Build history of the part. All positions in model axes, mm. A direction names the side the tool comes from. Give positions to 0.01 mm unless a question says otherwise; leave off trailing zeros. Loops run counter-clockwise (first coordinate to the right, second up) from the corner with the lowest first, then second, coordinate; pieces in that order, holes last. Notation, with made-up numbers: M -35,52.5 L -13,52.5 A35 cw -13,85.5 Z; hole C 67.25,-39 d10. An arc over 180 degrees is marked long. Answer in a Markdown table with one row per item. Add a question column.
```python
from build123d import *

# Parameters (mm, degrees)
BOSS_EXTRUDE1_DEPTH       = 40
REVOLVE1_START            = -44.95139953
REVOLVE1_OUTLINE_R        = 13.5
REVOLVE1_DEPTH            = 30.829897511
M18_CLEARANCE_HOLE1_D     = 20
M18_CLEARANCE_HOLE1_DEPTH = 25
SKETCH9_W                 = 1.6
SKETCH9_H                 = 27
CUT_EXTRUDE4_DEPTH        = 76.299241718
CUT_EXTRUDE4_DEPTH_BACK   = 76.299241718
SKETCH18_R                = 1.6
SCALE2_SCALE              = 1.25
SKETCH19_W                = 57
SKETCH19_H                = 20
CUT_EXTRUDE5_DEPTH        = 39
SKETCH20_W                = 40
SKETCH20_H                = 20
CUT_EXTRUDE6_DEPTH        = 10
SKETCH21_R                = 5.5
CUT_EXTRUDE7_DEPTH        = 96.0605556
SKETCH22_W                = 7.783449774
SKETCH22_H                = 2
SKETCH22_W_2              = 10.366550226
CUT_EXTRUDE8_DEPTH        = 2
SKETCH23_W                = 9.71853625
SKETCH23_H                = 7.281011564
CUT_EXTRUDE9_DEPTH        = 20
SKETCH25_W                = 2.5
SKETCH25_H                = 9
BOSS_EXTRUDE3_DEPTH       = 10
SKETCH26_W                = 2.5
SKETCH26_H                = 2
BOSS_EXTRUDE4_DEPTH       = 8
SKETCH27_R                = 2.1
CUT_EXTRUDE10_DEPTH       = 8
BOSS_EXTRUDE5_DEPTH       = 2
BOSS_EXTRUDE6_DEPTH       = 2


with BuildPart() as part:
    # Sketch1 → Boss-Extrude1 (new body)
    with BuildSketch(Plane(origin=(0, 40, 0), x_dir=(1, 0, 0), z_dir=(0, 1, 0))):
        with BuildLine():
            Line((-5.61521172, 20.235350191), (-42.5, 10))
            Line((-42.5, 10), (-42.5, -10))
            Line((-42.5, -10), (-5.61521172, -20.235350191))
            ThreePointArc((-5.61521172, -20.235350191), (21, 0), (-5.61521172, 20.235350191))
        make_face()
    extrude(amount=-BOSS_EXTRUDE1_DEPTH)

    # Revolve1: read off the stored shape, not the designer's step
    # Revolve1 outline → Revolve1 (add)
    with BuildSketch(Plane(origin=(0, 0, 0), x_dir=(0.9799247046208294, -0.02083962380947531, -0.19827577601224947), z_dir=(0.19936793441719802, 0.10243002349202102, 0.9745565745577031)).offset(REVOLVE1_START)):
        with Locations((-1.9070974, 22.005607966)):
            Circle(REVOLVE1_OUTLINE_R)
    extrude(amount=REVOLVE1_DEPTH)

    # M18 Clearance Hole1
    with Locations(Plane(origin=(-8.961867673, -4.60437291, -43.807681948), x_dir=(-0.9799247046208296, 0.02083962380947534, 0.19827577601224922), z_dir=(-0.19936793441719777, -0.10243002349202121, -0.9745565745577032))):
        with Locations((1.9070974, 22.005607966)):
            Hole(M18_CLEARANCE_HOLE1_D / 2, depth=M18_CLEARANCE_HOLE1_DEPTH)

    # Sketch9 → M3.5 Clearance Hole1 (revolve, cut)
    with BuildSketch(Plane(origin=(-18.009225855, 18.806465846, -31.591069121), x_dir=(-0.12392681772022805, 0.7153744254872676, -0.6876638533531477), z_dir=(0.1561720753640579, 0.6984304843277114, 0.6984304843277114))):
        with Locations((0.8, 13.5)):
            Rectangle(SKETCH9_W, SKETCH9_H)
    revolve(axis=Axis((-11.78670398, 18.674134235, -32.850120299), (-0.9799247046208297, 0.020839623809475325, 0.19827577601224802)), mode=Mode.SUBTRACT)

    # Sketch18 → Cut-Extrude4 (cut, two sides: drawn at the far end of the back side and taken through both)
    with BuildSketch(Plane(origin=(-1.740210315, 0.03700828, 0.352110268), x_dir=(-0.19823095447813932, 0.004215689735382395, -0.9801462730872066), z_dir=(0.9799247046208297, -0.020839623809475356, -0.19827577601224802)).offset(-CUT_EXTRUDE4_DEPTH_BACK)):
        with Locations(Location((34.613136918, 18.419306886, 0), (0, 0, 359.758405588))):
            Circle(SKETCH18_R)
    extrude(amount=CUT_EXTRUDE4_DEPTH + CUT_EXTRUDE4_DEPTH_BACK, mode=Mode.SUBTRACT)


with BuildPart() as part_1:
    # Scale2: scaled about (0, 0, 0)
    add(part.part.scale(SCALE2_SCALE))

    # Sketch19 → Cut-Extrude5 (cut)
    with BuildSketch(Plane(origin=(0, 50, 0), x_dir=(1, 0, 0), z_dir=(0, 1, 0))):
        with Locations((-11.2875, 0)):
            Rectangle(SKETCH19_W, SKETCH19_H)
    extrude(amount=-CUT_EXTRUDE5_DEPTH, mode=Mode.SUBTRACT)

    # Sketch20 → Cut-Extrude6 (cut)
    with BuildSketch(Plane(origin=(0, 11, 0), x_dir=(1, 0, 0), z_dir=(0, 1, 0))):
        with Locations((-13.154050226, 0)):
            Rectangle(SKETCH20_W, SKETCH20_H)
    extrude(amount=-CUT_EXTRUDE6_DEPTH, mode=Mode.SUBTRACT)

    # Sketch21 → Cut-Extrude7 (cut, through all)
    with BuildSketch(Plane.XZ):
        with Locations(Location((0, 0, 0), (0, 0, 270))):
            Circle(SKETCH21_R)
    extrude(amount=-CUT_EXTRUDE7_DEPTH, mode=Mode.SUBTRACT)

    # Sketch22 → Cut-Extrude8 (cut)
    with BuildSketch(Plane(origin=(0, 11, 0), x_dir=(1, 0, 0), z_dir=(0, 1, 0))):
        with Locations((-37.045775113, 0)):
            Rectangle(SKETCH22_W, SKETCH22_H)
        with Locations((12.029224887, 0)):
            Rectangle(SKETCH22_W_2, SKETCH22_H)
    extrude(amount=-CUT_EXTRUDE8_DEPTH, mode=Mode.SUBTRACT)

    # Sketch23 → Cut-Extrude9 (cut)
    with BuildSketch(Plane(origin=(0, 50, 0), x_dir=(1, 0, 0), z_dir=(0, 1, 0))):
        with Locations((22.071768125, 0)):
            Rectangle(SKETCH23_W, SKETCH23_H)
    extrude(amount=-CUT_EXTRUDE9_DEPTH, mode=Mode.SUBTRACT)

    # Sketch25 → Boss-Extrude3 (add)
    with BuildSketch(Plane(origin=(0, 1, 0), x_dir=(1, 0, 0), z_dir=(0, 1, 0))):
        with Locations((-31.904050226, 5.5)):
            Rectangle(SKETCH25_W, SKETCH25_H)
        with Locations((-31.904050226, -5.5)):
            Rectangle(SKETCH25_W, SKETCH25_H)
    extrude(amount=BOSS_EXTRUDE3_DEPTH)

    # Sketch26 → Boss-Extrude4 (add)
    with BuildSketch(Plane(origin=(0, 1, 0), x_dir=(1, 0, 0), z_dir=(0, 1, 0))):
        with Locations((-31.904050226, 0)):
            Rectangle(SKETCH26_W, SKETCH26_H)
    extrude(amount=BOSS_EXTRUDE4_DEPTH)

    # Sketch27 → Cut-Extrude10 (cut)
    with BuildSketch(Plane(origin=(0, 11, 0), x_dir=(1, 0, 0), z_dir=(0, 1, 0))):
        with Locations(Location((14.75, 4.85, 0), (0, 0, 270))):
            Circle(SKETCH27_R)
        with Locations(Location((14.75, -4.85, 0), (0, 0, 270))):
            Circle(SKETCH27_R)
        with Locations(Location((-34.75, 4.85, 0), (0, 0, 270))):
            Circle(SKETCH27_R)
        with Locations(Location((-34.75, -4.85, 0), (0, 0, 270))):
            Circle(SKETCH27_R)
    extrude(amount=-CUT_EXTRUDE10_DEPTH, mode=Mode.SUBTRACT)

    # Sketch35 → Boss-Extrude5 (add)
    with BuildSketch(Plane.XZ):
        with BuildLine():
            Line((-2.5, 7.071067812), (-2.5, 5.454356057))
            ThreePointArc((-2.5, 5.454356057), (0, 6), (2.5, 5.454356057))
            Line((2.5, 5.454356057), (2.5, 7.071067812))
            ThreePointArc((2.5, 7.071067812), (0, 7.5), (-2.5, 7.071067812))
        make_face()
    extrude(amount=BOSS_EXTRUDE5_DEPTH)

    # Sketch36 → Boss-Extrude6 (add)
    with BuildSketch(Plane.XZ.offset(2)):
        with BuildLine():
            Line((-2.5, 5.454356057), (-2.5, 11.42978565))
            ThreePointArc((-2.5, 11.42978565), (0, 11.7), (2.5, 11.42978565))
            Line((2.5, 11.42978565), (2.5, 5.454356057))
            ThreePointArc((2.5, 5.454356057), (0, 6), (-2.5, 5.454356057))
        make_face()
    extrude(amount=BOSS_EXTRUDE6_DEPTH)


solid = part_1.part
```
(1) Slice it at C-C, the plane x = 0. State how many separate pieces and enclosed holes the cut face has, then the cut area to 3 significant figures.
(2) Slice it at D-D, the plane x = -34.75. Give the cut face in (y, z).
(3) Tool access for faces 4 (the flat face through (-24.64, 15.75, -54.27)), 5 (the flat face through (-7.48, 25.03, -26.69)), 6 (the flat face through (-35.3, 11, 7.4)), 7 (the flat face through (22, 40, -3.641)): list every direction of +Z, -Z, +X, -X, +Y, -Y with a clear straight run to the whole face (end or side of a thin tool).
(4) Wall check: line 1 (X direction, y = 1.5, z = 1) (3 decimals); line 2 (X direction, y = 26.5, z = -8) (1 decimal); line 3 (X direction, y = 7, z = 4) (3 decimals). Give the ranges that are in metal, low to high.
(5) Pin check, flat tips, straight feed: pin 1 (2.5 mm diameter, centred on x = 14, z = -3.5, fed in from +Y); pin 2 (1.4 mm diameter, centred on x = 1, z = 9, fed in from +Y); pin 3 (4.5 mm diameter, centred on x = 20.5, y = 37.5, fed in from +Z). Stop position of each tip, or through.
(6) Slice it at B-B, the plane x = 14.75. Give the cut face in (y, z).
(7) Pull direction X, two halves, no side cores. Call faces 1 (the cylindrical face through (0, -2, 6)), 2 (the flat face through (-30.39, 25.35, 18.81)), 3 (the flat face through (0, -2, 9)): +X half, -X half, draft (parallel to the pull), parting line (faces both ways), or undercut.
Solution:
| question | item | result |
|---|---|---|
| 1 | separate pieces | 2 |
| 1 | enclosed holes | 1 |
| 1 | area | 2,170 mm^2 |
| 2 | outline | M 0,-17.6 L 50,-17.6 L 50,-10 L 11,-10 L 11,-6.95 L 3,-6.95 L 3,-2.75 L 11,-2.75 L 11,-1 L 9,-1 L 9,1 L 11,1 L 11,2.75 L 3,2.75 L 3,6.95 L 11,6.95 L 11,10 L 50,10 L 50,17.6 L 0,17.6 Z |
| 3 | face 4 | -Z, -X, -Y |
| 3 | face 5 | none |
| 3 | face 6 | +Y |
| 3 | face 7 | +X, +Y |
| 4 | line 1 | -53.125 to -30.654, 6.846 to 26.231 |
| 4 | line 2 | -53.1 to -39.8, 17.2 to 25 |
| 4 | line 3 | -53.125 to -36.67, -32.83 to -30.654, 6.846 to 12.83, 16.67 to 25.943 |
| 5 | pin 1 | y = 11 |
| 5 | pin 2 | y = 1 |
| 5 | pin 3 | z = 18.87 |
| 6 | outline | M 0,-21.71 L 50,-21.71 L 50,-10 L 11,-10 L 11,-6.95 L 3,-6.95 L 3,-2.75 L 11,-2.75 L 11,-1 L 9,-1 L 9,1 L 11,1 L 11,2.75 L 3,2.75 L 3,6.95 L 11,6.95 L 11,10 L 50,10 L 50,21.71 L 0,21.71 Z |
| 7 | face 1 | undercut |
| 7 | face 2 | -X half |
| 7 | face 3 | draft |
